Geometry check sheet. Reference: the model listing, model coordinates, mm. Face numbers are marked on the shaded views. A direction names the side the tool comes from. Round coordinates to 2 decimals unless told otherwise and drop trailing zeros. Write each loop counter-clockwise with the first axis right and the second up, starting at its lowest first coordinate (ties: lowest second). Pieces come first, ordered by that corner, then holes.
Autodesk Fusion 360 part; units mm, degrees
sketch "Sketch1" plane through (0, 0, 0) normal (0, 0, 1) x (1, 0, 0)
  line L0 (0, 0) -> (275, 0)
  line L1 (275, 0) -> (275, -165)
  line L2 (275, -165) -> (0, -165)
  line L3 (0, -165) -> (0, 0)
  dimension "d1" = 275
  dimension "d2" = 165
extrude "Extrude1" add sketch "Sketch1" along normal blind 5
sketch "Sketch2" plane through (0, 0, 5) normal (0, 0, 1) x (-1, 0, 0)
  line L0 (0, 165) -> (-275, 165)
  line L1 (-275, 165) -> (-275, 0)
  line L2 (-275, 0) -> (0, 0)
  line L3 (0, 0) -> (0, 165)
  line L4 (0, 0) -> (-275, 0)
  line L5 (-275, 0) -> (-275, 5)
  line L6 (-275, 5) -> (0, 5)
  line L7 (0, 5) -> (0, 0)
  line L8 (-275, 0) -> (-270, 0)
  line L9 (-270, 0) -> (-270, 165)
  line L10 (-270, 165) -> (-275, 165)
  line L11 (-275, 165) -> (-275, 0)
  line L12 (-275, 165) -> (0, 165)
  line L13 (0, 165) -> (0, 160)
  line L14 (0, 160) -> (-275, 160)
  line L15 (-275, 160) -> (-275, 165)
  line L16 (0, 0) -> (-5, 0)
  line L17 (-5, 0) -> (-5, 165)
  line L18 (-5, 165) -> (0, 165)
  line L19 (0, 165) -> (0, 0)
  dimension "d5" = 5
  dimension "d6" = 5
  dimension "d7" = 165
  dimension "d8" = 275
  dimension "d9" = 5
  dimension "d10" = 165
sketch "Sketch3" plane through (0, 0, 5) normal (0, 0, 1) x (-1, 0, 0)
extrude "Extrude2" add sketch "Sketch2" along normal blind 150 contours L0 L3 L12 L13 L14 L17 L18 L19 | L3 L6 L14 L17 L19 | L2 L3 L4 L6 L7 L16 L17 L19
sketch "Sketch4" plane through (0, 0, 5) normal (0, 0, 1) x (-1, 0, 0)
  line L0 (-5, 0) -> (-5, 165)
  line L1 (-5, 165) -> (-275, 165)
  line L2 (-275, 165) -> (-275, 0)
  line L3 (-275, 0) -> (-5, 0)
sketch "Sketch5" plane through (0, 0, 5) normal (0, 0, 1) x (-1, 0, 0)
  line L0 (-275, 0) -> (-270, 0)
  line L1 (-270, 0) -> (-270, 165)
  line L2 (-270, 165) -> (-275, 165)
  line L3 (-275, 165) -> (-275, 0)
  line L4 (-5, 0) -> (-5, 165)
  dimension "d13" = 5
  dimension "d14" = 165
  dimension "d15" = 270
extrude "Extrude3" add sketch "Sketch5" along normal blind 150
sketch "Sketch6" plane through (0, 0, 0) normal (0, 1, 0) x (1, 0, 0)
  line L0 (269.7146, -155) -> (269.7146, -150)
  line L1 (4.7146, -150) -> (4.7146, -155)
  line L2 (5, -5) -> (275, -5)
  dimension "d19" = 5
sketch "Sketch7" plane through (0, 0, 5) normal (0, 0, 1) x (-1, 0, 0)
  curve L0
  curve L1
  curve L2
  curve L3
  line L4 (-275, 165) -> (-275, 160)
  line L5 (-275, 165) -> (-275, 160)
  line L6 (-5, 160) -> (-5, 165)
  line L7 (-5, 0) -> (-275, 0)
  dimension "d21" = 265
  dimension "d22" = 5
  dimension "d25" = 270
  dimension "d26" = 145
  dimension "d27" = 265
sketch "Sketch8" plane through (0, 0, 0) normal (0, 1, 0) x (1, 0, 0)
  line L0 (5.2103, -149.946) -> (270.2103, -149.946)
  line L1 (5, -5) -> (275, -5)
sketch "Sketch9" plane through (0, 0, 5) normal (0, 0, 1) x (1, 0, 0)
sketch "Sketch10" plane through (275, 0, 0) normal (1, 0, 0) x (0, 1, 0)
  line L0 (-165, 0) -> (0, 0)
  line L1 (0, 0) -> (0, 155)
  line L2 (0, 155) -> (-165, 155)
  line L3 (-165, 155) -> (-165, 0)
  line L4 (-165, 155) -> (0, 155)
  line L5 (0, 155) -> (0, 150)
  line L6 (0, 150) -> (-165, 150)
  line L7 (-165, 150) -> (-165, 155)
  dimension "d29" = 165
  dimension "d30" = 5
extrude "Extrude4" add sketch "Sketch10" against normal blind 275 contours L1 L2 L3 L4 L5 L6 L7
sketch "Sketch11" plane through (0, 0, 0) normal (0, 1, 0) x (1, 0, 0)
sketch "Sketch12" plane through (0, 0, 0) normal (0, 1, 0) x (1, 0, 0)
sketch "Sketch13" plane through (275, 0, 0) normal (1, 0, 0) x (0, 1, 0)
  line L0 (-165, 155) -> (-165, 0)
  line L1 (-165, 0) -> (0, 0)
  line L2 (0, 0) -> (0, 155)
  line L3 (0, 155) -> (-165, 155)
  line L4 (-165, 155) -> (-135, 155) construction
sketch "Sketch14" plane through (275, 0, 0) normal (1, 0, 0) x (0, 1, 0)
  line L0 (-170, 155) -> (-5, 155)
  line L1 (-5, 155) -> (-5, 225)
  line L2 (-5, 225) -> (-170, 225)
  line L3 (-170, 225) -> (-170, 155)
  line L4 (-165, 5) -> (0, 5)
  line L5 (-170, 155) -> (-87.1175, 224.5467)
  line L6 (-170, 155) -> (-61.8046, 155) construction
  line L7 (-87.1175, 224.5467) -> (13.9338, 144.1668)
  line L8 (-87.1175, 224.5467) -> (42.0037, 224.5467) construction
  dimension "d35" = 165
  dimension "d36" = 70
  dimension "d37" = 150
  dimension "d38" = 40
  dimension "d39" = 38.5
extrude "Extrude5" add sketch "Sketch14" against normal blind 5 contours L0 L1 L5 L7
sketch "Sketch15" plane through (0, 0, 155) normal (0, 0, 1) x (-1, 0, 0)
  line L0 (-270, 5) -> (-275, 5)
  line L1 (-275, 5) -> (-275, 0)
  line L2 (-275, 0) -> (0, 0)
  line L3 (0, 0) -> (0, 165)
  line L4 (0, 165) -> (-270, 165)
  line L5 (-270, 165) -> (-270, 5)
sketch "Sketch16" plane through (0, 0, 0) normal (-1, 0, 0) x (0, -1, 0)
  line L0 (0, 155) -> (0, 0)
  line L1 (0, 0) -> (165, 0)
  line L2 (165, 0) -> (165, 155)
  line L3 (165, 155) -> (0, 155)
  line L4 (0, 155) -> (87.0576, 225.2184)
  line L5 (87.0576, 225.2184) -> (165, 159.0254)
  line L6 (165, 159.0254) -> (165, 155)
extrude "Extrude6" add sketch "Sketch16" against normal blind 5 contours L3 L4 L5 L6
sketch "Sketch17" plane through (5, 0, 0) normal (1, 0, 0) x (0, 1, 0)
  line L0 (-87.0576, 225.2184) -> (-165, 159.0254)
  line L1 (-165, 159.0254) -> (-165, 155)
  line L2 (-165, 155) -> (0, 155)
  line L3 (0, 155) -> (-87.0576, 225.2184)
sketch "Sketch18" plane through (0, 0, 0) normal (0, 1, 0) x (1, 0, 0)
  curve L0
  curve L1
  curve L2
  curve L3
  dimension "d44" = 265
  dimension "d45" = 5
sketch "Sketch19" plane through (275, 0, 0) normal (1, 0, 0) x (0, 1, 0)
  line L0 (-165, 155) -> (-165, 0)
  line L1 (-165, 0) -> (0, 0)
  line L2 (0, 0) -> (0, 155)
  line L3 (0, 155) -> (-5, 155)
  line L4 (-5, 155) -> (-5, 159.2275)
  line L5 (-5, 159.2275) -> (-87.1175, 224.5467)
  line L6 (-87.1175, 224.5467) -> (-170, 155)
  line L7 (-170, 155) -> (-165, 155)
  line L8 (-165, 155) -> (-87, 220)
  line L9 (-87, 220) -> (-46.1419, 187.5)
  line L10 (-46.1419, 187.5) -> (-5, 155)
sketch "Sketch20" plane through (0, 0, 155) normal (0, 0, 1) x (-1, 0, 0)
  circle A0 centre (-75, 123.9573) radius 32.5
  line L0 (-270, 165) -> (-270, 5)
  line L1 (-270.2103, 3.9573) -> (-5.2104, 3.9572)
  dimension "d46" = 65
  dimension "d47" = 195
  dimension "d48" = 120
extrude "Extrude7" cut sketch "Sketch20" against normal blind 5
sketch "Sketch21" plane through (275, 0, 0) normal (1, 0, 0) x (0, 1, 0)
sketch "Sketch22" plane through (5, 0, 0) normal (1, 0, 0) x (0, 1, 0)
extrude "Extrude8" cut sketch "Sketch19" against normal blind 150 contours L4 L5 L6 L7 L8 L9 L10
sketch "Sketch23" plane through (0, 0, 0) normal (0, 1, 0) x (1, 0, 0)
equation "d1 = 165 mm + 65 mm + 35 mm + 10 mm"
equation "d2 = 55 mm + 48 mm + 10 mm + 52 mm"
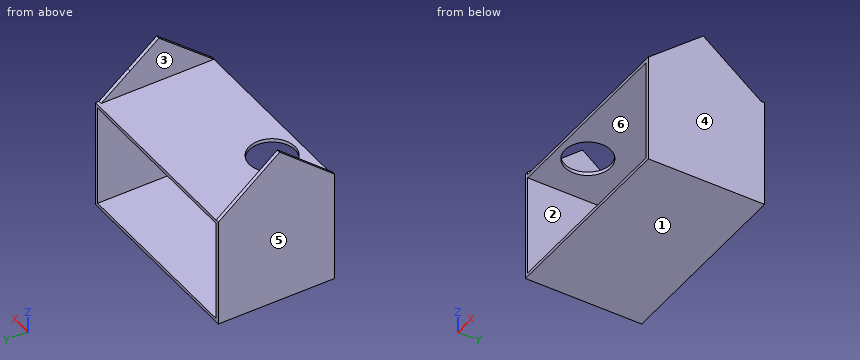
1. Section check A-A (x = 75). Record the cut outline in (y, z).
2. Section check C-C (x = 18). Record the cut outline in (y, z), plus the area to 3 significant figures.
3. Access from +Z, -Z, +X, -X, +Y, -Y to the whole of each face (thin tool, end or side, straight path). Record for the marked faces 1, 2 and 3.
4. Section check D-D (y = -41). Record the cut outline in (x, z).
5. Depth check by flat-ended pin: pin 1 Ø4 at (x, y) = (45, -30) entering from +Z. Enter the tip coordinate at first touch or a pass-through.
6. Release check for a two-part mould opening along X. For the marked faces 4, 5 and 6 record: +X half, -X half, draft (parallel to the pull), parting line (faces both ways), or undercut.
7. Section check B-B (z = 82). Record the cut outline in (x, y).
8. Scan lines: line 1 along Z through (x, y) = (29.5, -48.5); line 2 along X through (y, z) = (-6.5, 149.5); line 3 along Y through (x, z) = (75, 151.25). Record each from-to range of solid material in increasing order.
Results below:
1. outline: (-165, 0) - (0, 0) - (0, 5) - (-165, 5) - close; (-165, 150) - (-156.46, 150) - (-156.46, 155) - (-165, 155) - close; (-91.46, 150) - (0, 150) - (0, 155) - (-91.46, 155) - close
2. outline: (-165, 0) - (0, 0) - (0, 5) - (-165, 5) - close; (-165, 150) - (0, 150) - (0, 155) - (-165, 155) - close
2. area: 1,650 mm2
3. face 1: -Z, +X, -X, +Y, -Y
3. face 2: +Y, -Y
3. face 3: +Z, +Y, -Y
4. outline: (0, 0) - (275, 0) - (275, 183.44) - (270, 183.44) - (270, 155) - (5, 155) - (5, 188.07) - (0, 188.07) - close; hole (5, 5) - (270, 5) - (270, 150) - (5, 150) - close
5. pin 1: stops at z = 155
6. face 4: +X half
6. face 5: -X half
6. face 6: undercut
7. outline: (0, -165) - (5, -165) - (5, 0) - (0, 0) - close; (270, -165) - (275, -165) - (275, 0) - (270, 0) - close
8. line 1: z = 0 to 5, 150 to 155
8. line 2: x = 0 to 5, 270 to 275
8. line 3: y = -165 to -156.46, -91.46 to 0
